Read the model definition and answer for the solid it produces. Units are mm, in the model's axes. Face numbers are marked on the shaded views. A direction names the side the tool comes from. Give positions to 0.01 mm unless a question says otherwise; leave off trailing zeros. Loops run counter-clockwise (first coordinate to the right, second up) from the corner with the lowest first, then second, coordinate; pieces in that order, holes last. Notation, with made-up numbers: (47, 83) - (61, 83) arc R33 cw to (61, 121) - close; hole circle Ø1 at (76.25, 39.25). An arc over 180 degrees is marked (long way). Use a Markdown table: item, result. Add a question column.
Item 1: A cutting plane is placed at C-C (y = 102). Determine the outline of the cut face in (x, z).
Item 2: A cutting plane is placed at B-B (x = -178). Determine the outline of the cut face in (y, z), plus the area to 3 significant figures.
Item 3: Which of the six approach directions +Z, -Z, +X, -X, +Y, -Y give full straight-line access (tool end or side, diameter ignored) to the marked faces 4, 5, 6 and 7?
Item 4: This flat-tipped pin is pushed along its axis until it touches: P1, Ø5.5, axis at x = -180.5, y = 125, coming from the +Z side. Where does it stop, or does it pass through?
Item 5: Consider probe 1 along X at (y, z) = (115, 13.35); probe 2 along Y at (x, z) = (-180, 14.4); probe 3 along Y at (x, z) = (-183.75, 11.4). Determine where each line is inside the solid, lowest interval first. Write a range as [from, to].
Item 6: For a pull along X with two mould halves and no side action, classify the marked faces 1, 2 and 3 as +X half, -X half, draft (parallel to the pull), parting line (faces both ways), or undercut.
Item 7: A cutting plane is placed at A-A (z = 13.9). Determine the outline of the cut face in (x, y).
Item 8: A cutting plane is placed at D-D (z = 12.25). Determine the outline of the cut face in (x, y), plus the area to 3 significant figures.
from build123d import *

# Parameters (mm, degrees)
SKETCH1_W           = 12.3
SKETCH1_H           = 32.5
SKETCH1_R           = 1
BOSS_EXTRUDE1_DEPTH = 3
FILLET1_R           = 1.2
FILLET2_R           = 6
SKETCH2_W           = 12.3
SKETCH2_H           = 27.5
BOSS_EXTRUDE2_DEPTH = 2.5
FILLET3_R           = 6
SKETCH3_W           = 6
SKETCH3_H           = 4
CUT_EXTRUDE1_DEPTH  = 227.640270134
CUT_EXTRUDE2_DEPTH  = 2.5
SKETCH5_R           = 2.75
CUT_EXTRUDE3_DEPTH  = 227.593384825


with BuildPart() as part:
    # Sketch1 → Boss-Extrude1 (new body)
    with BuildSketch(Plane.XY.offset(10)):
        with Locations((-182.01249108, 109.965842893)):
            Rectangle(SKETCH1_W, SKETCH1_H)
        with Locations((-185.999386631, 123.827694148)):
            Circle(SKETCH1_R, mode=Mode.SUBTRACT)
        with Locations((-177.999386631, 123.827694148)):
            Circle(SKETCH1_R, mode=Mode.SUBTRACT)
    extrude(amount=BOSS_EXTRUDE1_DEPTH)

    # Fillet1
    fillet1_edges = [part.edges().sort_by_distance(p)[0] for p in [
        (-188.16249108, 126.215842893, 11.5),
        (-175.86249108, 126.215842893, 11.5),
    ]]
    fillet(fillet1_edges, radius=FILLET1_R)

    # Fillet2
    fillet2_edges = [part.edges().sort_by_distance(p)[0] for p in [
        (-175.86249108, 93.715842893, 11.5),
        (-188.16249108, 93.715842893, 11.5),
    ]]
    fillet(fillet2_edges, radius=FILLET2_R)

    # Sketch2 → Boss-Extrude2 (add)
    with BuildSketch(Plane.XY.offset(13)):
        with Locations((-182.01249108, 107.27562942)):
            Rectangle(SKETCH2_W, SKETCH2_H)
    extrude(amount=BOSS_EXTRUDE2_DEPTH)

    # Fillet3
    fillet3_edges = [part.edges().sort_by_distance(p)[0] for p in [
        (-188.16249108, 93.52562942, 14.25),
        (-175.86249108, 93.52562942, 14.25),
    ]]
    fillet(fillet3_edges, radius=FILLET3_R)

    # Sketch3 → Cut-Extrude1 (cut, through all)
    with BuildSketch(Plane.XY.offset(15.5)):
        with Locations((-181.88348906, 116.80293228)):
            Rectangle(SKETCH3_W, SKETCH3_H)
    extrude(amount=-CUT_EXTRUDE1_DEPTH, mode=Mode.SUBTRACT)

    # Sketch4 → Cut-Extrude2 (cut)
    with BuildSketch(Plane.XY.offset(15.5)):
        with BuildLine():
            Line((-184.138427734, 113.48600769), (-179.861572266, 113.48600769))
            Line((-179.861572266, 113.48600769), (-178.824890137, 99.586959839))
            ThreePointArc((-178.824890137, 99.586959839), (-181.83374979, 96.789675787), (-185.116622925, 99.259651184))
            Line((-185.116622925, 99.259651184), (-184.138427734, 113.48600769))
        make_face()
    extrude(amount=-CUT_EXTRUDE2_DEPTH, mode=Mode.SUBTRACT)

    # Sketch5 → Cut-Extrude3 (cut, through all)
    with BuildSketch(Plane.XY.offset(13)):
        with Locations((-182.06249108, 99.972659898)):
            Circle(SKETCH5_R)
    extrude(amount=-CUT_EXTRUDE3_DEPTH, mode=Mode.SUBTRACT)


solid = part.part
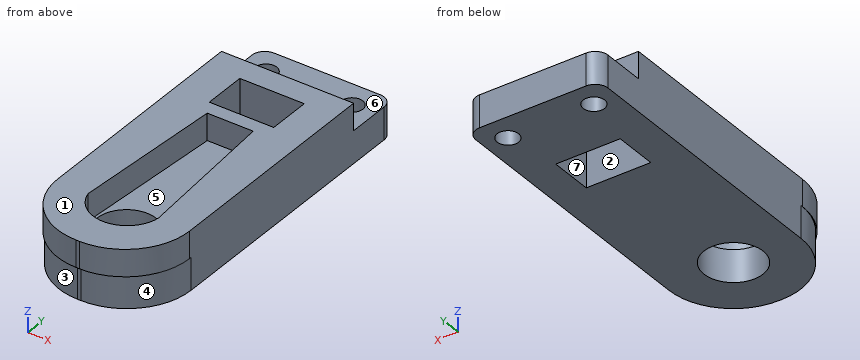
Geometry says:
| question | item | result |
|---|---|---|
| 1 | outline | (-188.16, 10) - (-183.92, 10) - (-183.92, 13) - (-184.93, 13) - (-184.93, 15.5) - (-188.16, 15.5) - close; (-180.2, 10) - (-175.86, 10) - (-175.86, 15.5) - (-179, 15.5) - (-179, 13) - (-180.2, 13) - close |
| 2 | outline | (94.93, 13) - (95.12, 13) - (95.12, 10) - (122.83, 10) - (122.83, 13) - (121.03, 13) - (121.03, 15.5) - (94.93, 15.5) - close; (124.83, 10) - (126.22, 10) - (126.22, 13) - (124.83, 13) - close |
| 2 | area | 153 mm² |
| 3 | face 4 | -Z, +X, -Y |
| 3 | face 5 | +Z |
| 3 | face 6 | +Z, +X, -X, +Y |
| 3 | face 7 | +Z, -Z |
| 4 | P1 | z = 13 |
| 5 | probe 1 | [-188.16, -184.88], [-178.88, -175.86] |
| 5 | probe 2 | [93.82, 97.49], [113.49, 114.8], [118.8, 121.03] |
| 5 | probe 3 | [93.93, 97.8], [102.14, 114.8], [118.8, 126.22] |
| 6 | face 1 | draft |
| 6 | face 2 | undercut |
| 6 | face 3 | -X half |
| 7 | outline | (-188.16, 99.53) arc R6 ccw to (-182.16, 93.53) - (-181.86, 93.53) arc R6 ccw to (-175.86, 99.53) - (-175.86, 121.03) - (-188.16, 121.03) - close; hole (-185.12, 99.26) arc R3.2 ccw to (-178.82, 99.59) - (-179.86, 113.49) - (-184.14, 113.49) - close; hole (-184.88, 114.8) - (-178.88, 114.8) - (-178.88, 118.8) - (-184.88, 118.8) - close |
| 8 | outline | (-188.16, 99.72) arc R6 ccw to (-182.16, 93.72) - (-181.86, 93.72) arc R6 ccw to (-175.86, 99.72) - (-175.86, 125.02) arc R1.2 ccw to (-177.06, 126.22) - (-186.96, 126.22) arc R1.2 ccw to (-188.16, 125.02) - close; hole circle Ø2 at (-186, 123.83); hole (-184.88, 114.8) - (-178.88, 114.8) - (-178.88, 118.8) - (-184.88, 118.8) - close; hole circle Ø5.5 at (-182.06, 99.97); hole circle Ø2 at (-178, 123.83) |
| 8 | area | 330 mm² |
